Geometry check sheet. Reference: drawing and pictorial views, mm from the part's lowest x, y, z. A direction names the side the tool comes from. Round coordinates to 2 decimals unless told otherwise and drop trailing zeros. Write each loop counter-clockwise with the first axis right and the second up, starting at its lowest first coordinate (ties: lowest second). Pieces come first, ordered by that corner, then holes.
Item 1: Depth check by flat-ended pin: pin 1 (0.9 mm diameter, centred on x = 5, y = 2, fed in from +Z). Enter the tip coordinate at first touch or a pass-through.
Item 2: Section check A-A, the plane y = 1.15. Record the cut outline in (x, z).
Item 3: Release check for a two-part mould opening along Y. For the marked faces 3, 4, 5 and 6 record: pulls with the +Y half, pulls with the -Y half, needs draft (parallel to the pull), parting line crosses it, or undercut.
Item 4: Section check C-C, the plane y = 2.4. Record the cut outline in (x, z).
Item 5: Section check D-D, the plane z = 1.85. Record the cut outline in (x, y).
Item 6: Material ranges on line 1 along Z through (x, y) = (0.35, 1.5); line 2 along X through (y, z) = (0.9, 2.15), recorded low to high.
Item 7: Section check B-B, the plane z = 1.15. Record the cut outline in (x, y), plus the area to 3 significant figures.
Item 8: Set-up check for the marked faces 1 and 2: record each of +Z, -Z, +X, -X, +Y, -Y from which the full face is reachable in a straight line by a thin tool's end or side.
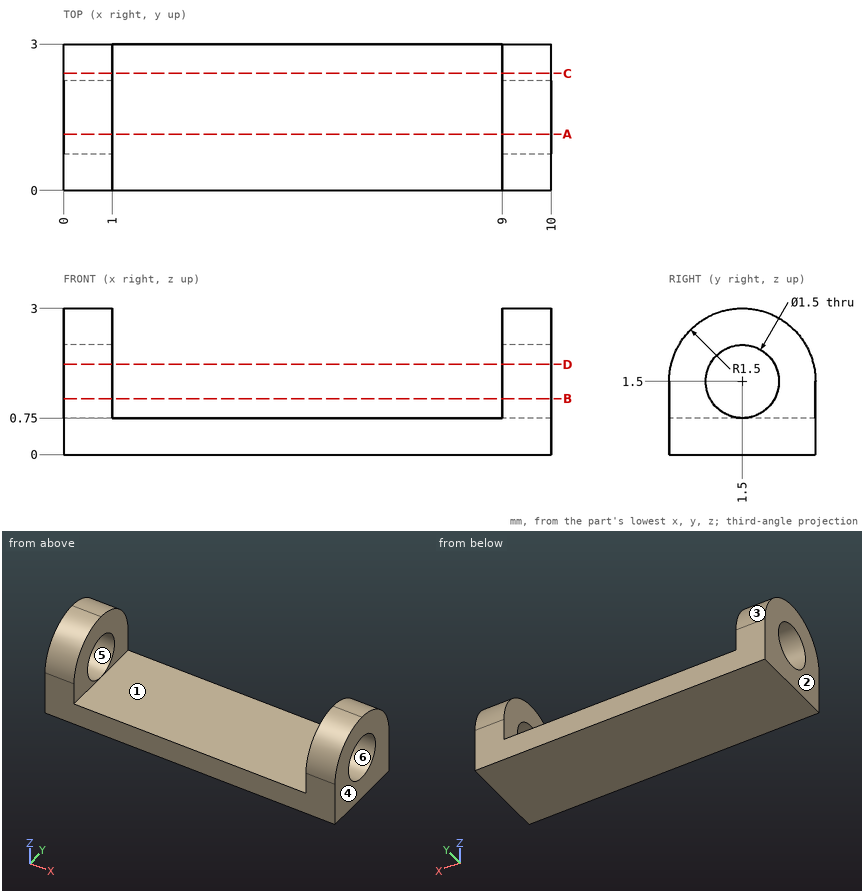
Values found:
1. pin 1: stops at z = 0.75
2. outline: (0, 0) - (10, 0) - (10, 0.84) - (9, 0.84) - (9, 0.75) - (1, 0.75) - (1, 0.84) - (0, 0.84) - close; (0, 2.16) - (1, 2.16) - (1, 2.96) - (0, 2.96) - close; (9, 2.16) - (10, 2.16) - (10, 2.96) - (9, 2.96) - close
3. face 3: pulls with the +Y half
3. face 4: needs draft
3. face 5: undercut
3. face 6: undercut
4. outline: (0, 0) - (10, 0) - (10, 2.7) - (9, 2.7) - (9, 0.75) - (1, 0.75) - (1, 2.7) - (0, 2.7) - close
5. outline: (0, 0.04) - (1, 0.04) - (1, 0.84) - (0, 0.84) - close; (0, 2.16) - (1, 2.16) - (1, 2.96) - (0, 2.96) - close; (9, 0.04) - (10, 0.04) - (10, 0.84) - (9, 0.84) - close; (9, 2.16) - (10, 2.16) - (10, 2.96) - (9, 2.96) - close
6. line 1: z = 0 to 0.75, 2.25 to 3
6. line 2: x = 0 to 1, 9 to 10
7. outline: (0, 0) - (1, 0) - (1, 0.84) - (0, 0.84) - close; (0, 2.16) - (1, 2.16) - (1, 3) - (0, 3) - close; (9, 0) - (10, 0) - (10, 0.84) - (9, 0.84) - close; (9, 2.16) - (10, 2.16) - (10, 3) - (9, 3) - close
7. area: 3.35 mm2
8. face 1: +Z, +Y, -Y
8. face 2: +Z, -Z, -X, +Y, -Y
